Read the model definition and answer for the solid it produces. Units are mm, in the model's axes. A direction names the side the tool comes from. Coordinates: 2 decimals unless noted, no trailing zeros. Loops run counter-clockwise (first coordinate to the right, second up) from the corner with the lowest first, then second, coordinate; pieces in that order, holes last. Notation, with made-up numbers: (34.25, 28) - (66.25, 28) arc R28 ccw to (66.25, 46) - close; hole circle Ø7 at (-16.5, -10). An arc over 180 degrees is marked (long way). One line per question, with ' | ' between items. Start each with the question number.
```python
from build123d import *

# Parameters (mm, degrees)
F0_R     = 5
F0_W     = 20
F0_H     = 20
F1_DEPTH = 50


with BuildPart() as f1:
    # F0 (on Top) → F1 (new body)
    with BuildSketch(Plane.XY):
        with BuildLine():
            Line((-16.160254, 216.968965), (-195.980762, -94.489292))
            ThreePointArc((-195.980762, -94.489292), (-195.980762, -113.149546), (-179.820508, -122.479673))
            Line((-179.820508, -122.479673), (179.820508, -122.479673))
            ThreePointArc((179.820508, -122.479673), (195.980762, -113.149546), (195.980762, -94.489292))
            Line((195.980762, -94.489292), (16.160254, 216.968965))
            ThreePointArc((16.160254, 216.968965), (0, 226.299092), (-16.160254, 216.968965))
        make_face()
        Polygon((-167.5, -85.159165), (-157.5, -102.479673), (-174.820508, -112.479673), (-184.820508, -95.159165), align=None, mode=Mode.SUBTRACT)
        Circle(F0_R, mode=Mode.SUBTRACT)
        Polygon((157.5, -102.479673), (167.5, -85.159165), (184.820508, -95.159165), (174.820508, -112.479673), align=None, mode=Mode.SUBTRACT)
        with Locations((0, 197.638837)):
            Rectangle(F0_W, F0_H, mode=Mode.SUBTRACT)
    extrude(amount=F1_DEPTH)


solid = f1.part
```
1) Which of the six approach directions +Z, -Z, +X, -X, +Y, -Y give full straight-line access (tool end or side, diameter ignored) to faces 1 (the cylindrical face through (-196.116, -112.912, 24.65)), 2 (the flat face through (162.43, -93.94, 24.65))?
2) The part is cut by section B-B on x = 0. Write down the section's boundary in (y, z).
3) Given pin 1 Ø6 at (y, z) = (199.5, 21.5) entering from +X; pin 2 Ø13 at (x, y) = (0, 0) entering from +Z; pin 3 Ø1 at (x, z) = (-132, 24) entering from +Y; pin 4 Ø1 at (y, z) = (22.5, 9) entering from -X, each flat-ended and moving along its own axis, determine where each tip first touches the part or whether it passes through.
4) The mould has two halves that part along X. Classify faces 3 (the flat face through (107.33, 59.06, 24.65)), 4 (the flat face through (-179.75, -103.94, 24.65)), 5 (the cylindrical face through (0.274, 226.297, 24.65)): released by +X, released by -X, zero draft, split by the parting line, or undercut.
5) The part is cut by section C-C on y = 0. Write down the section's boundary in (x, z), and give its area (3 significant figures).
6) Find the intervals of material crossed by line 1 along Y through (x, z) = (0, 26); line 2 along X through (y, z) = (198.5, 23.5); line 3 along X through (y, z) = (199, 43), in increasing order. Write a range as from..to.
7) The part is cut by section D-D on y = 158.5. Write down the section's boundary in (x, z), and give its area (3 significant figures).
8) The part is cut by section A-A on z = 18. Write down the section's boundary in (x, y).
Answer below:
1) face 1: +Z, -Z, -X | face 2: +Z, -Z
2) outline: (-122.48, 0) - (-5, 0) - (-5, 50) - (-122.48, 50) - close; (5, 0) - (187.64, 0) - (187.64, 50) - (5, 50) - close; (207.64, 0) - (226.3, 0) - (226.3, 50) - (207.64, 50) - close
3) pin 1: x = 27.98 | pin 2: z = 50 | pin 3: y = 17.19 | pin 4: x = -128.73
4) face 3: released by +X | face 4: undercut | face 5: split by the parting line
5) outline: (-141.43, 0) - (-5, 0) - (-5, 50) - (-141.43, 50) - close; (5, 0) - (141.43, 0) - (141.43, 50) - (5, 50) - close | area: 13,600 mm2
6) line 1: -122.48..-5, 5..187.64, 207.64..226.3 | line 2: -26.82..-10, 10..26.82 | line 3: -26.53..-10, 10..26.53
7) outline: (-49.92, 0) - (49.92, 0) - (49.92, 50) - (-49.92, 50) - close | area: 4,990 mm2
8) outline: (-195.98, -94.49) arc R18.66 ccw to (-179.82, -122.48) - (179.82, -122.48) arc R18.66 ccw to (195.98, -94.49) - (16.16, 216.97) arc R18.66 ccw to (-16.16, 216.97) - close; hole (-184.82, -95.16) - (-174.82, -112.48) - (-157.5, -102.48) - (-167.5, -85.16) - close; hole (-10, 187.64) - (10, 187.64) - (10, 207.64) - (-10, 207.64) - close; hole circle Ø10 at (0, 0); hole (157.5, -102.48) - (174.82, -112.48) - (184.82, -95.16) - (167.5, -85.16) - close
